The listing builds one solid part. Answer for the finished solid, in the listing's coordinates (mm). Face numbers are marked on the shaded views. Coordinates: 2 decimals unless noted, no trailing zeros. Order: outer loops, then holes, each group sorted by start corner. A loop starts at its lowest first (then second) coordinate and runs counter-clockwise, first axis right, second up. Notation, with made-up numbers: (-12.75, 60) -> (38.25, 60) arc R30 ccw to (38.25, 92) -> close; hole circle Ø7 at (26.5, 68.5). An arc over 180 degrees is marked (long way). Return JSON: item names as keys, results as strings.
```python
from build123d import *

# Parameters (mm, degrees)
SKETCH1_R           = 19.05
SKETCH1_R_2         = 1.27
SKETCH1_R_3         = 4.7625
BOSS_EXTRUDE1_DEPTH = 3.175


with BuildPart() as part:
    # Sketch1 → Boss-Extrude1 (new body)
    with BuildSketch(Plane.XY):
        Circle(SKETCH1_R)
        with Locations((0, 15.875)):
            Circle(SKETCH1_R_2, mode=Mode.SUBTRACT)
        with Locations((11.225320151, 11.225320151)):
            Circle(SKETCH1_R_2, mode=Mode.SUBTRACT)
        with Locations((15.875, 0)):
            Circle(SKETCH1_R_2, mode=Mode.SUBTRACT)
        Circle(SKETCH1_R_3, mode=Mode.SUBTRACT)
        with Locations((11.225320151, -11.225320151)):
            Circle(SKETCH1_R_2, mode=Mode.SUBTRACT)
        with Locations((0, -15.875)):
            Circle(SKETCH1_R_2, mode=Mode.SUBTRACT)
        with Locations((-11.225320151, -11.225320151)):
            Circle(SKETCH1_R_2, mode=Mode.SUBTRACT)
        with Locations((-15.875, 0)):
            Circle(SKETCH1_R_2, mode=Mode.SUBTRACT)
        with Locations((-11.225320151, 11.225320151)):
            Circle(SKETCH1_R_2, mode=Mode.SUBTRACT)
    extrude(amount=BOSS_EXTRUDE1_DEPTH)


solid = part.part
```
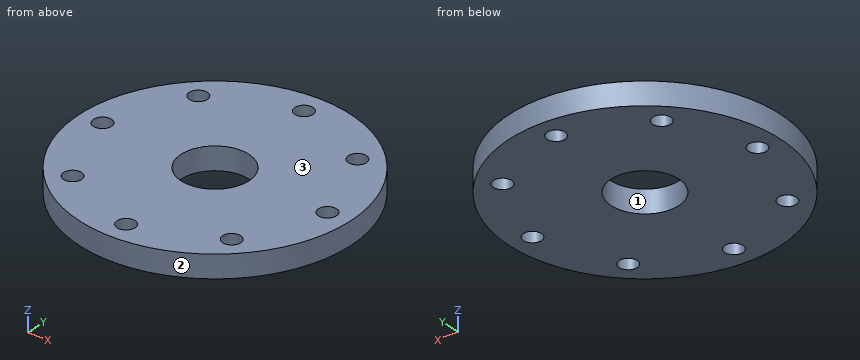
Item 1: Find the intervals of material crossed by probe 1 along X at (y, z) = (12, 1.2); probe 2 along Y at (x, z) = (10.5, 2.1); probe 3 along Y at (x, z) = (1, 0.35), in increasing order.
Answer list:
{"probe 1": "-14.8 to -12.23, -10.22 to 10.22, 12.23 to 14.8", "probe 2": "-15.9 to -12.27, -10.18 to 10.18, 12.27 to 15.9", "probe 3": "-19.02 to -16.66, -15.09 to -4.66, 4.66 to 15.09, 16.66 to 19.02"}
Item 2: Determine the mould class of the marked faces 1, 2 and 3 for opening direction X: pulls with the +X half, pulls with the -X half, needs draft (parallel to the pull), parting line crosses it, or undercut.
Answer list:
{"face 1": "undercut", "face 2": "parting line crosses it", "face 3": "needs draft"}
Item 3: Flat-ended cylindrical pins translate along their axes: pin 1 (2 mm diameter, centred on x = 15.875, y = 0, fed in from -Z); pin 2 (1 mm diameter, centred on x = -1, z = 0.5, fed in from -Y); pin 3 (1.5 mm diameter, centred on y = 11, z = 1, fed in from -X). Find the tip coordinate at first contact, or state that the pin passes through.
Answer list:
{"pin 1": "through", "pin 2": "y = -19.04", "pin 3": "x = -16.06"}
Item 4: The part is cut by section A-A on y = 0. Count the separate pieces of the cut face and the enclosed holes in it, plus the area to 3 significant figures.
Answer list:
{"separate pieces": "4", "enclosed holes": "0", "area": "74.6 mm2"}
Item 5: The part is cut by section C-C on x = -16.5. Determine the outline of the cut face in (y, z) (3 decimals), plus the area to 3 significant figures.
Answer list:
{"outline": "(-9.521, 0) -> (-1.106, 0) -> (-1.106, 3.175) -> (-9.521, 3.175) -> close; (1.106, 0) -> (9.521, 0) -> (9.521, 3.175) -> (1.106, 3.175) -> close", "area": "53.4 mm2"}
